Here's how the part is built. I have some questions about the finished solid (model axes, mm). Face numbers are marked on the shaded views. A direction names the side the tool comes from. Round coordinates to 2 decimals unless told otherwise and drop trailing zeros. Order: outer loops, then holes, each group sorted by start corner. A loop starts at its lowest first (then second) coordinate and runs counter-clockwise, first axis right, second up. Notation, with made-up numbers: (58, 3.25) - (96, 3.25) arc R25 ccw to (96, 31.25) - close; hole circle Ø10 at (-24, 83). An arc over 180 degrees is marked (long way). One line per item, written item: value.
from build123d import *

# Parameters (mm, degrees)
F0_R     = 11.0236
F1_DEPTH = 6.35
F3_DEPTH = 6.35


with BuildPart() as f1:
    # F0 (on Top) → F1 (new body)
    with BuildSketch(Plane.XY):
        Polygon((0, -57.15), (24.7466759131, -14.2875), (-24.7466759131, -14.2875), align=None)
        Polygon((-4.5827177617, -36.5125), (-9.1654355234, -28.575), (-4.5827177617, -20.6375), (4.5827177617, -20.6375), (9.1654355234, -28.575), (4.5827177617, -36.5125), align=None, mode=Mode.SUBTRACT)
        Polygon((-24.7466759131, -14.2875), (24.7466759131, -14.2875), (0, 28.575), align=None)
        Circle(F0_R, mode=Mode.SUBTRACT)
        Polygon((0, 28.575), (24.7466759131, -14.2875), (49.4933518263, 28.575), align=None)
        Polygon((33.9121114365, 14.2875), (29.3293936748, 6.35), (20.1639581514, 6.35), (15.5812403898, 14.2875), (20.1639581514, 22.225), (29.3293936748, 22.225), align=None, mode=Mode.SUBTRACT)
        Polygon((-49.4933518263, 28.575), (-24.7466759131, -14.2875), (0, 28.575), align=None)
        Polygon((-20.1639581514, 22.225), (-15.5812403898, 14.2875), (-20.1639581514, 6.35), (-29.3293936748, 6.35), (-33.9121114365, 14.2875), (-29.3293936748, 22.225), align=None, mode=Mode.SUBTRACT)
    extrude(amount=F1_DEPTH)

    # F2 (on face) → F3 (cut)
    with BuildSketch(Plane.XY.offset(6.35)):
        Polygon((6.5991135768, 28.575), (-6.5991135768, 28.575), (0, 17.145), align=None)
        Polygon((-14.8480055479, -8.5725), (-28.0462327016, -8.5725), (-21.4471191247, -20.0025), align=None)
        Polygon((21.4471191247, -20.0025), (28.0462327016, -8.5725), (14.8480055479, -8.5725), align=None)
    extrude(amount=-F3_DEPTH, mode=Mode.SUBTRACT)


solid = f1.part
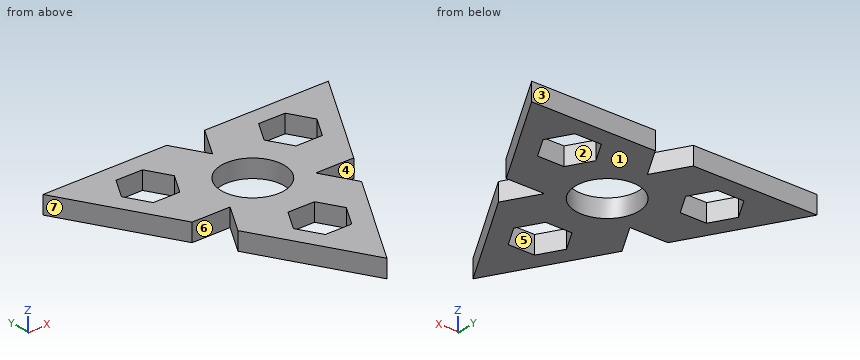
Q1. If we section it at B-B, the plane y = 13: Please give me the cut outline in (x, z).
Results list:
outline: (-40.5, 0) - (-33.17, 0) - (-33.17, 6.35) - (-40.5, 6.35) - close; (-16.32, 0) - (16.32, 0) - (16.32, 6.35) - (-16.32, 6.35) - close; (33.17, 0) - (40.5, 0) - (40.5, 6.35) - (33.17, 6.35) - close
Q2. If we section it at D-D, the plane x = 13.5: Please give me the cut outline in (y, z) (3 decimals).
Results list:
outline: (-33.767, 0) - (28.575, 0) - (28.575, 6.35) - (-33.767, 6.35) - close
Q3. If I drill on line 1 along Y through (x, z) = (-18.5, 3.75) (1 decimal); line 2 along X through (y, z) = (-27, 3.25); line 3 along X through (y, z) = (13.5, 0.75), over which ranges is the centre line in solid material (lowest first)?
Results list:
line 1: -25.1 to -14.9, -8.6 to 9.2, 19.3 to 28.6
line 2: -17.41 to -8.26, 8.26 to 17.41
line 3: -40.79 to -33.46, -16.04 to 16.04, 33.46 to 40.79
Q4. Which directions (+Z, -Z, +X, -X, +Y, -Y) give clear straight access to the entire face, cutting with the end or side of a thin tool? Please do the marked faces 4, 5, 6 and 7.
Results list:
face 4: +Z, -Z, +X
face 5: +Z, -Z
face 6: +Z, -Z, -X
face 7: +Z, -Z, -X, -Y
Q5. If we section it at C-C, the plane y = 0: Please give me the cut outline in (x, z).
Results list:
outline: (-33, 0) - (-11.02, 0) - (-11.02, 6.35) - (-33, 6.35) - close; (11.02, 0) - (33, 0) - (33, 6.35) - (11.02, 6.35) - close
Q6. Will these pins go through, and if not, where does the flat tip stop? pin 1 (1.9 mm diameter, centred on x = -22.5, z = 3, fed in from -Y); pin 2 (3 mm diameter, centred on y = -32.5, z = 1, fed in from +X); pin 3 (5 mm diameter, centred on x = -1, y = 9.5, fed in from -Z); pin 4 (3 mm diameter, centred on x = -20.5, z = 3.5, fed in from -Y).
Results list:
pin 1: y = -8.57
pin 2: x = 15.1
pin 3: z = 0
pin 4: y = -24.24
Q7. We'd pull the mould along Y, two halves only. Please class the marked faces 1, 2 and 3: released by +Y, released by -Y, zero draft, split by the parting line, or undercut.
Results list:
face 1: zero draft
face 2: undercut
face 3: released by +Y
